```python
from build123d import *

# Parameters (mm, degrees)
SKETCH1_W           = 36
SKETCH1_H           = 20
BOSS_EXTRUDE1_DEPTH = 1.9
BOSS_EXTRUDE2_DEPTH = 1.9
SKETCH5_W           = 59.232531926
SKETCH5_H           = 32.087665796
CUT_EXTRUDE2_DEPTH  = 10
SKETCH10_R          = 1.75
CUT_EXTRUDE3_DEPTH  = 10
SKETCH11_R          = 1.6
CUT_EXTRUDE4_DEPTH  = 4


with BuildPart() as part:
    # Sketch1 → Boss-Extrude1 (new body)
    with BuildSketch(Plane(origin=(0, 0, 0), x_dir=(1, 0, 0), z_dir=(0, 1, 0))):
        Rectangle(SKETCH1_W, SKETCH1_H)
    extrude(amount=BOSS_EXTRUDE1_DEPTH)

    # Sketch5 → Cut-Extrude2 (cut)
    with BuildSketch(Plane(origin=(0, 1.9, 0), x_dir=(1, 0, 0), z_dir=(0, 1, 0))):
        Rectangle(SKETCH5_W, SKETCH5_H)
    extrude(amount=-CUT_EXTRUDE2_DEPTH, mode=Mode.SUBTRACT)


with BuildPart() as body_2:
    # Sketch3 → Boss-Extrude2 (new body)
    with BuildSketch(Plane.XZ):
        with BuildLine():
            Line((-37.576725301, 45.574302205), (-37.576725301, 56.574302205))
            Line((-37.576725301, 56.574302205), (-13.576725301, 56.574302205))
            Line((-13.576725301, 56.574302205), (-13.576725301, 40.574302205))
            Line((-13.576725301, 40.574302205), (13.576725301, 40.574302205))
            Line((13.576725301, 40.574302205), (13.576725301, 56.574302205))
            Line((13.576725301, 56.574302205), (37.576725301, 56.574302205))
            Line((37.576725301, 56.574302205), (37.576725301, 45.574302205))
            Line((37.576725301, 45.574302205), (63.576725301, 45.574302205))
            ThreePointArc((63.576725301, 45.574302205), (0, 92.574302205), (-63.576725301, 45.574302205))
            Line((-63.576725301, 45.574302205), (-37.576725301, 45.574302205))
        make_face()
    extrude(amount=-BOSS_EXTRUDE2_DEPTH)

    # Sketch10 → Cut-Extrude3 (cut)
    with BuildSketch(Plane(origin=(0, 1.9, 0), x_dir=(1, 0, 0), z_dir=(0, 1, 0))):
        with Locations((-12.5, -88.074302205)):
            Circle(SKETCH10_R)
        with Locations((12.5, -88.074302205)):
            Circle(SKETCH10_R)
        with Locations((0, -63.074302205)):
            Circle(SKETCH10_R)
    extrude(amount=-CUT_EXTRUDE3_DEPTH, mode=Mode.SUBTRACT)

    # Sketch11 → Cut-Extrude4 (cut)
    with BuildSketch(Plane.XZ):
        with Locations((-55, 51.074302205)):
            Circle(SKETCH11_R)
        with Locations((55, 51.074302205)):
            Circle(SKETCH11_R)
    extrude(amount=-CUT_EXTRUDE4_DEPTH, mode=Mode.SUBTRACT)


solid = body_2.part
```
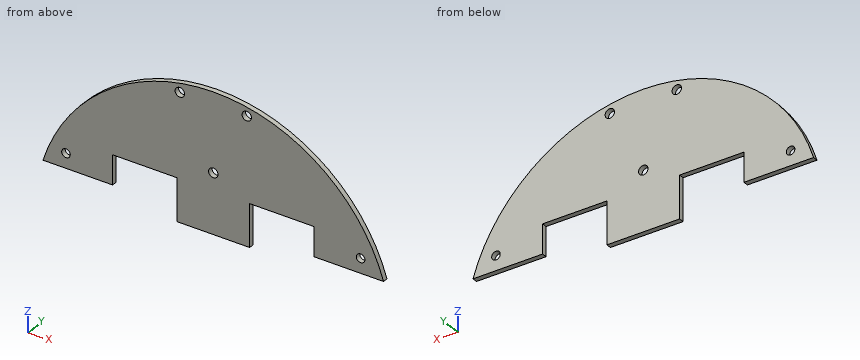
Read the model definition and answer for the solid it produces. Units are mm, in the model's axes. Coordinates: 2 decimals unless noted, no trailing zeros. Write each loop counter-clockwise with the first axis right and the second up, starting at its lowest first coordinate (ties: lowest second). Pieces come first, ordered by that corner, then holes. Notation, with made-up numbers: (37, 46) - (51, 46) arc R22 cw to (51, 80) - close; hole circle Ø9 at (72.25, 86.5). An arc over 180 degrees is marked (long way). Answer as a JSON object with one key per item and string values. Group by question number.
1. A cutting plane is placed at A-A (x = 0). Determine the outline of the cut face in (y, z).
2. A cutting plane is placed at B-B (z = 54). Determine the outline of the cut face in (x, y), plus the area to 3 significant figures.
3. Consider L1, parallel to Z at x = 0, y = 1; L2, parallel to X at y = 0.4, z = 46; L3, parallel to X at y = 1.1, z = 48.5. Determine where each line is inside the solid, lowest interval first. Write a range as [from, to].
4. Each of these flat-tipped pins is pushed along its axis until it touches: P1, Ø1, axis at x = -27, y = 1.5, coming from the -Z side; P2, Ø1, axis at y = 1.5, z = 73, coming from the +X side; P3, Ø0.6, axis at x = -44.5, y = 1, coming from the -Z side. Where does it stop, or does it pass through?
5. A cutting plane is placed at C-C (y = 1.5). Determine the outline of the cut face in (x, z), plus the area to 3 significant figures.
6. A cutting plane is placed at D-D (x = 55). Determine the outline of the cut face in (y, z), plus the area to 3 significant figures.
Worked out:
{
 "1": {"outline": "(0, 40.57) - (1.9, 40.57) - (1.9, 61.32) - (0, 61.32) - close; (0, 64.82) - (1.9, 64.82) - (1.9, 92.57) - (0, 92.57) - close"},
 "2": {"outline": "(-60.35, 0) - (-37.58, 0) - (-37.58, 1.9) - (-60.35, 1.9) - close; (-13.58, 0) - (13.58, 0) - (13.58, 1.9) - (-13.58, 1.9) - close; (37.58, 0) - (60.35, 0) - (60.35, 1.9) - (37.58, 1.9) - close", "area": "138 mm²"},
 "3": {"L1": "z = [40.57, 61.32], [64.82, 92.57]", "L2": "x = [-63.44, -37.58], [-13.58, 13.58], [37.58, 63.44]", "L3": "x = [-62.6, -37.58], [-13.58, 13.58], [37.58, 62.6]"},
 "4": {"P1": "stops at z = 56.57", "P2": "stops at x = 47.61", "P3": "stops at z = 45.57"},
 "5": {"outline": "(-63.58, 45.57) - (-37.58, 45.57) - (-37.58, 56.57) - (-13.58, 56.57) - (-13.58, 40.57) - (13.58, 40.57) - (13.58, 56.57) - (37.58, 56.57) - (37.58, 45.57) - (63.58, 45.57) arc R66.5 ccw to start; hole circle Ø3.2 at (-55, 51.07); hole circle Ø3.5 at (-12.5, 88.07); hole circle Ø3.5 at (0, 63.07); hole circle Ø3.5 at (12.5, 88.07); hole circle Ø3.2 at (55, 51.07)", "area": "3,950 mm²"},
 "6": {"outline": "(0, 45.57) - (1.9, 45.57) - (1.9, 49.47) - (0, 49.47) - close; (0, 52.67) - (1.9, 52.67) - (1.9, 63.45) - (0, 63.45) - close", "area": "27.9 mm²"}
}
